Source: CAD feature listing. Evaluate the final solid. Frame: model axes, mm. Face numbers are marked on the shaded views. A direction names the side the tool comes from. Round coordinates to 2 decimals unless told otherwise and drop trailing zeros. Order: outer loops, then holes, each group sorted by start corner. A loop starts at its lowest first (then second) coordinate and runs counter-clockwise, first axis right, second up. Notation, with made-up numbers: (28, -17.5) - (59, -17.5) arc R7 ccw to (59, -13.5) - close; hole circle Ø3 at (82.5, 21.25). An arc over 180 degrees is marked (long way). Put each result on its own line as item: value. Start each with the question number.
1) Contact query for flat-ended pins moving along their axis: P1, Ø3, axis at y = 6.5, z = -2.5, coming from the -X side; P2, Ø3, axis at y = 5.5, z = 6, coming from the -X side. Output: stop coordinate, or through.
2) Section A-A on z = -4.5. Output: boundary loops of the cut face in (x, y).
3) Access query for the marked faces 1 and 2. Directions: +Z, -Z, +X, -X, +Y, -Y. A direction counts if a zero-diameter tool reaches every point of the face in a straight line with its end or side. Return the directions, or none.
4) Section B-B on x = 23. Output: boundary loops of the cut face in (y, z).
5) Section D-D on z = 33. Output: boundary loops of the cut face in (x, y), then the cut area to 3 significant figures.
6) Section C-C on y = 3.5. Output: boundary loops of the cut face in (x, z).
7) Line query: probe 1 along Y at (x, z) = (67, -5.5); probe 2 along Z at (x, y) = (10.5, 7); probe 3 along X at (y, z) = (4.5, 18). Output: solid intervals per line, ascending. Write a range as [from, to].
```python
from build123d import *

# Parameters (mm, degrees)
IZIM1_W                     = 101.194983934
IZIM1_H                     = 49.38315216
Y_KSEKLIK_EKSTR_ZYON2_DEPTH = 24
G_VDE_TA_KOPYALA1_ANGLE     = 90
IZIM2_R                     = 17.60947899
Y_KSEKLIK_EKSTR_ZYON4_DEPTH = 13


with BuildPart() as part:
    # Çizim1 → Yükseklik-Ekstrüzyon2 (new body)
    with BuildSketch(Plane.XY):
        with Locations((38.049313959, -10.524278329)):
            Rectangle(IZIM1_W, IZIM1_H)
    extrude(amount=Y_KSEKLIK_EKSTR_ZYON2_DEPTH)


with BuildPart() as part_1:
    # Gövde-Taşı/Kopyala1: moved
    add(part.part.rotate(Axis((0, -10.524278329, 12), (1, 0, 0)), G_VDE_TA_KOPYALA1_ANGLE))

    # Çizim2 → Yükseklik-Ekstrüzyon4 (add)
    with BuildSketch(Plane(origin=(0, 1.475721671, 0), x_dir=(1, 0, 0), z_dir=(0, 1, 0))):
        with Locations(Location((14.659162211, -10.95067627, 0), (0, 0, 90))):
            Circle(IZIM2_R)
    extrude(amount=Y_KSEKLIK_EKSTR_ZYON4_DEPTH)


solid = part_1.part
```
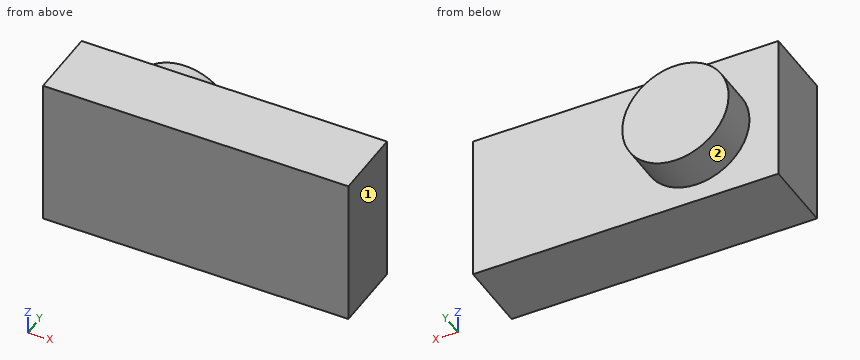
Answer sheet:
1. P1: x = 1.73
1. P2: x = -2.61
2. outline: (-12.55, -22.52) - (88.65, -22.52) - (88.65, 1.48) - (23.11, 1.48) - (23.11, 14.48) - (6.21, 14.48) - (6.21, 1.48) - (-12.55, 1.48) - close
3. face 1: +Z, -Z, +X, +Y, -Y
3. face 2: +Y
4. outline: (-22.52, -12.69) - (1.48, -12.69) - (1.48, -4.56) - (14.48, -4.56) - (14.48, 26.46) - (1.48, 26.46) - (1.48, 36.69) - (-22.52, 36.69) - close
5. outline: (-12.55, -22.52) - (88.65, -22.52) - (88.65, 1.48) - (-12.55, 1.48) - close
5. area: 2,430 mm^2
6. outline: circle Ø35.22 at (14.66, 10.95)
7. probe 1: [-22.52, 1.48]
7. probe 2: [-6.16, 28.06]
7. probe 3: [-1.48, 30.8]
